Here's how the part is built. I have some questions about the finished solid (model axes, mm). Round coordinates to 2 decimals unless told otherwise and drop trailing zeros. Order: outer loops, then holes, each group sorted by start corner. A loop starts at its lowest first (then second) coordinate and runs counter-clockwise, first axis right, second up. Notation, with made-up numbers: (3, 68.25) -> (38, 68.25) arc R24 ccw to (38, 95.25) -> close; hole circle Ø2 at (-14, 26.25). An arc over 180 degrees is marked (long way). Answer in a Markdown table with one row per item.
```python
from build123d import *

# Parameters (mm, degrees)
SKETCH1_W           = 50
SKETCH1_H           = 50
BOSS_EXTRUDE1_DEPTH = 1.5
SKETCH2_R           = 5.25
CUT_EXTRUDE1_DEPTH  = 3
FILLET1_R           = 6
SKETCH3_W           = 13
SKETCH3_H           = 24
CUT_EXTRUDE2_DEPTH  = 3


with BuildPart() as part:
    # Sketch1 → Boss-Extrude1 (new body, symmetric)
    with BuildSketch(Plane(origin=(0, 0, 0), x_dir=(1, 0, 0), z_dir=(0, 1, 0))):
        Rectangle(SKETCH1_W, SKETCH1_H)
    extrude(amount=BOSS_EXTRUDE1_DEPTH, both=True)

    # Sketch2 → Cut-Extrude1 (cut)
    with BuildSketch(Plane(origin=(0, 1.5, 0), x_dir=(1, 0, 0), z_dir=(0, 1, 0))):
        with Locations((17, -17)):
            Circle(SKETCH2_R)
        with Locations((-17, -17)):
            Circle(SKETCH2_R)
        with Locations((-17, 17)):
            Circle(SKETCH2_R)
        with Locations((17, 17)):
            Circle(SKETCH2_R)
    extrude(amount=-CUT_EXTRUDE1_DEPTH, mode=Mode.SUBTRACT)

    # Fillet1
    fillet1_edges = [part.edges().sort_by_distance(p)[0] for p in [
        (25, 0, 25),
        (-25, 0, 25),
        (-25, 0, -25),
        (25, 0, -25),
    ]]
    fillet(fillet1_edges, radius=FILLET1_R)

    # Sketch3 → Cut-Extrude2 (cut)
    with BuildSketch(Plane.XZ.offset(1.5)):
        Rectangle(SKETCH3_W, SKETCH3_H)
    extrude(amount=-CUT_EXTRUDE2_DEPTH, mode=Mode.SUBTRACT)


solid = part.part
```
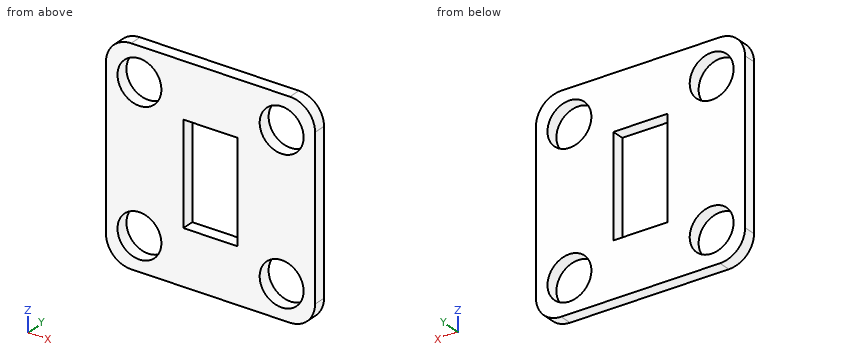
1. Suppose I cut it at B-B on x = -5.5. Write out the boundary of the cut face in (y, z), then the cut area to 3 significant figures.
Numbers:
| item | result |
|---|---|
| outline | (-1.5, -25) -> (1.5, -25) -> (1.5, -12) -> (-1.5, -12) -> close; (-1.5, 12) -> (1.5, 12) -> (1.5, 25) -> (-1.5, 25) -> close |
| area | 78.0 mm2 |
2. Please list where these lines run through material, in increasing order: line 1 along X through (y, z) = (-0.1, 17); line 2 along Z through (x, y) = (0.5, 0.15).
Numbers:
| item | result |
|---|---|
| line 1 | x = -25 to -22.25, -11.75 to 11.75, 22.25 to 25 |
| line 2 | z = -25 to -12, 12 to 25 |
3. Suppose I cut it at A-A on z = -17. Write out the boundary of the cut face in (x, y).
Numbers:
| item | result |
|---|---|
| outline | (-25, -1.5) -> (-22.25, -1.5) -> (-22.25, 1.5) -> (-25, 1.5) -> close; (-11.75, -1.5) -> (11.75, -1.5) -> (11.75, 1.5) -> (-11.75, 1.5) -> close; (22.25, -1.5) -> (25, -1.5) -> (25, 1.5) -> (22.25, 1.5) -> close |
4. Suppose I cut it at C-C on x = 17. Write out the boundary of the cut face in (y, z), then the cut area to 3 significant figures.
Numbers:
| item | result |
|---|---|
| outline | (-1.5, -25) -> (1.5, -25) -> (1.5, -22.25) -> (-1.5, -22.25) -> close; (-1.5, -11.75) -> (1.5, -11.75) -> (1.5, 11.75) -> (-1.5, 11.75) -> close; (-1.5, 22.25) -> (1.5, 22.25) -> (1.5, 25) -> (-1.5, 25) -> close |
| area | 87.0 mm2 |
5. Suppose I cut it at D-D on z = 11. Write out the boundary of the cut face in (x, y), then the cut area to 3 significant figures.
Numbers:
| item | result |
|---|---|
| outline | (-25, -1.5) -> (-6.5, -1.5) -> (-6.5, 1.5) -> (-25, 1.5) -> close; (6.5, -1.5) -> (25, -1.5) -> (25, 1.5) -> (6.5, 1.5) -> close |
| area | 111 mm2 |
